Read the model definition and answer for the solid it produces. Units are mm, in the model's axes. A direction names the side the tool comes from. Give positions to 0.01 mm unless a question says otherwise; leave off trailing zeros. Order: outer loops, then holes, each group sorted by start corner. A loop starts at its lowest first (then second) coordinate and runs counter-clockwise, first axis right, second up. Notation, with made-up numbers: M 40.5,35 L 62.5,35 A18 ccw 62.5,63 Z; hole C 67,88 d2. An arc over 180 degrees is marked long. Write item = value, one per line. Start each with the question number.
from build123d import *

# Parameters (mm, degrees)
SKETCH1_W                  = 47.625
SKETCH1_H                  = 25.4
BOSS_EXTRUDE1_DEPTH        = 9.525
SKETCH2_R                  = 6.757528855
BOSS_EXTRUDE2_DEPTH        = 25.4
BOSS_EXTRUDE3_DEPTH        = 25.4
F_8_0_199_DIAMETER_HOLE1_D = 5.0546
CHAMFER1_SIZE              = 3.175
CHAMFER2_SIZE              = 1.5875
F_8_0_199_DIAMETER_HOLE2_D = 5.0546
CUT_EXTRUDE1_REACH         = 714.11
SKETCH11_R                 = 6.35


with BuildPart() as part:
    # Sketch1 → Boss-Extrude1 (new body)
    with BuildSketch(Plane.XY):
        with Locations((-14.2875, 698.230229864)):
            Rectangle(SKETCH1_W, SKETCH1_H)
    extrude(amount=BOSS_EXTRUDE1_DEPTH)



with BuildPart() as body_2:
    # Sketch2 → Boss-Extrude2 (new body)
    with BuildSketch(Plane(origin=(0, 710.930229864, 0), x_dir=(-1, 0, 0), z_dir=(0, -1, 0))):
        with Locations(Location((-8.061541228, -17.843768092, 0), (0, 0, 270))):
            Circle(SKETCH2_R)
    extrude(amount=BOSS_EXTRUDE2_DEPTH)


with BuildPart() as part_1:
    add(part.part)

    add(body_2.part)  # Boss-Extrude3 merges body 2
    # Sketch3 → Boss-Extrude3 (add)
    with BuildSketch(Plane.XZ.offset(-685.530229864)):
        with BuildLine():
            Line((9.525, 9.525), (-7.01475572, 9.525))
            ThreePointArc((-7.01475572, 9.525), (-1.132498391, 11.961510763), (1.304012372, 17.843768092))
            ThreePointArc((1.304012372, 17.843768092), (4.433439084, 12.142797029), (10.923230214, 11.722090841))
            ThreePointArc((10.923230214, 11.722090841), (9.904202194, 10.827138231), (9.525, 9.525))
        make_face()
    extrude(amount=-BOSS_EXTRUDE3_DEPTH)

    # #8 (0.199) Diameter Hole1 (through all)
    with Locations(Plane(origin=(0, 710.930229864, 0), x_dir=(1, 0, 0), z_dir=(0, 1, 0))):
        with Locations((8.061541228, -17.843768092)):
            f_8_0_199_diameter_hole1 = Hole(F_8_0_199_DIAMETER_HOLE1_D / 2)

    # Chamfer1
    chamfer1_edges = [part_1.edges().sort_by_distance(p)[0] for p in [
        (-38.1, 710.930229864, 4.7625),
        (-38.1, 685.530229864, 4.7625),
    ]]
    chamfer(chamfer1_edges, length=CHAMFER1_SIZE)

    # Chamfer2
    chamfer2_edges = [part_1.edges().sort_by_distance(p)[0] for p in [
        (-20.96987786, 710.930229864, 9.525),
        (9.904202194, 685.530229864, 10.827138231),
        (-1.132498391, 685.530229864, 11.961510763),
        (9.904202194, 710.930229864, 10.827138231),
        (-1.132498391, 710.930229864, 11.961510763),
        (11.689643371, 685.530229864, 23.544739156),
        (11.689643371, 710.930229864, 23.544739156),
        (-20.96987786, 685.530229864, 9.525),
        (-38.1, 698.230229864, 9.525),
        (-36.5125, 709.342729864, 9.525),
        (-36.5125, 687.117729864, 9.525),
        (9.525, 710.930229864, 4.7625),
        (9.525, 685.530229864, 4.7625),
    ]]
    chamfer(chamfer2_edges, length=CHAMFER2_SIZE)

    # Mirror2: #8 (0.199) Diameter Hole1 across plane
    add(f_8_0_199_diameter_hole1.mirror(Plane.ZX.offset(698.230229864)), mode=Mode.SUBTRACT)

    # #8 (0.199) Diameter Hole2 (through all)
    with Locations(Plane(origin=(0, 0, 0), x_dir=(-1, 0, 0), z_dir=(0, 0, -1))):
        with Locations((9.525, 698.230229864), (28.575, 698.230229864)):
            Hole(F_8_0_199_DIAMETER_HOLE2_D / 2)

    # Sketch11 → Cut-Extrude1 (cut, up to next)
    with BuildSketch(Plane.XY.offset(9.525), mode=Mode.PRIVATE) as cut_extrude1_sk1:
        with Locations((-9.525, 698.230229864)):
            Circle(SKETCH11_R)
    cut_extrude1_tool1 = extrude(cut_extrude1_sk1.sketch, amount=CUT_EXTRUDE1_REACH, mode=Mode.PRIVATE) & part_1.part
    add(cut_extrude1_tool1.solids().sort_by_distance((-9.525, 698.23023, 9.525))[0], mode=Mode.SUBTRACT)


solid = part_1.part
1) Find section B-B on y = 690.75. Determine the outline of the cut face in (x, z) (1 decimal).
2) Each of these flat-tipped pins is pushed along its axis until it touches: P1, Ø8, axis at y = 697.5, z = 12.5, coming from the -X side; P2, Ø3, axis at y = 699, z = 5, coming from the +X side (3 decimals); P3, Ø2, axis at y = 707, z = 20, coming from the +X side. Where does it stop, or does it pass through?
3) Find section A-A on y = 696.25. Determine the outline of the cut face in (x, z) (1 decimal).
4) For a pull along Y with two mould halves and no side action, classify faces 5 (the face through (-27.409, 695.988, 4.829)), 6 (the face through (-21.165, 686.335, 8.742)), 7 (the face through (11.859, 698.386, 23.434)), 8 (the face through (-3.176, 698.127, 9.884)) as pulls with the +Y half, pulls with the -Y half, needs draft (parallel to the pull), parting line crosses it, or undercut.
5) Find section D-D on z = 4.25. Determine the outline of the cut face in (x, y) (1 decimal), plus the area to 3 significant figures.
6) For faces 1 (the face through (8.72, 710.15, 4.83)), 2 (the face through (-36.535, 687.14, 3.913)), 3 (the face through (9.525, 698, 5)), 4 (the face through (-21.17, 710.15, 8.72)), determine the directions among +Z, -Z, +X, -X, +Y, -Y from which every point of the face is accessible in a straight line to the end or side of a thin tool.
7) Find the intervals of material crossed by probe 1 along X at (y, z) = (687.75, 18); probe 2 along Z at (x, y) = (-5.5, 701) (3 decimals); probe 3 along X at (y, z) = (691.5, 18.5), in increasing order. Write a range as [from, to].
8) Find section C-C on x = -30. Determine the outline of the cut face in (y, z) (1 decimal).
Numbers:
q1.outline = M -38.1,0 L 9.5,0 L 9.5,9.5 A2.4 cw 10.9,11.7 A6.8 ccw long 1.3,17.8 A8.3 cw -7,9.5 L -36.5,9.5 L -38.1,7.9 Z; hole C 8.1,17.8 d5.1
q2.P1 = -37.54
q2.P2 = 9.525
q2.P3 = 14.72
q3.outline = M -38.1,0 L -30.1,0 L -30.1,9.5 L -36.5,9.5 L -38.1,7.9 Z; M -27,0 L -11.1,0 L -11.1,9.5 L -27,9.5 Z; M -8,0 L 9.5,0 L 9.5,9.5 A2.4 cw 10.9,11.7 A6.8 ccw long 1.3,17.8 A8.3 cw -3.5,10.3 L -3.5,9.5 L -8,9.5 Z; hole C 8.1,17.8 d5.1
q4.face_5 = undercut
q4.face_6 = pulls with the -Y half
q4.face_7 = needs draft
q4.face_8 = undercut
q5.outline = M -38.1,688.7 L -34.9,685.5 L 7.9,685.5 L 9.5,687.1 L 9.5,709.3 L 7.9,710.9 L -34.9,710.9 L -38.1,707.8 Z; hole C -28.6,698.2 d5.1; hole C -9.5,698.2 d5.1
q5.area = 1,160 mm2
q6.face_1 = -Z, +X, +Y
q6.face_2 = +Z, -Z, -X, -Y
q6.face_3 = -Z, +X, +Y, -Y
q6.face_4 = +Z, -X, +Y
q7.probe_1 = [1.31, 5.54], [10.58, 14.82]
q7.probe_2 = [0, 9.525]
q7.probe_3 = [1.34, 5.62], [10.5, 14.79]
q8.outline = M 685.5,0 L 696.1,0 L 696.1,9.5 L 687.1,9.5 L 685.5,7.9 Z; M 700.3,0 L 710.9,0 L 710.9,7.9 L 709.3,9.5 L 700.3,9.5 Z
